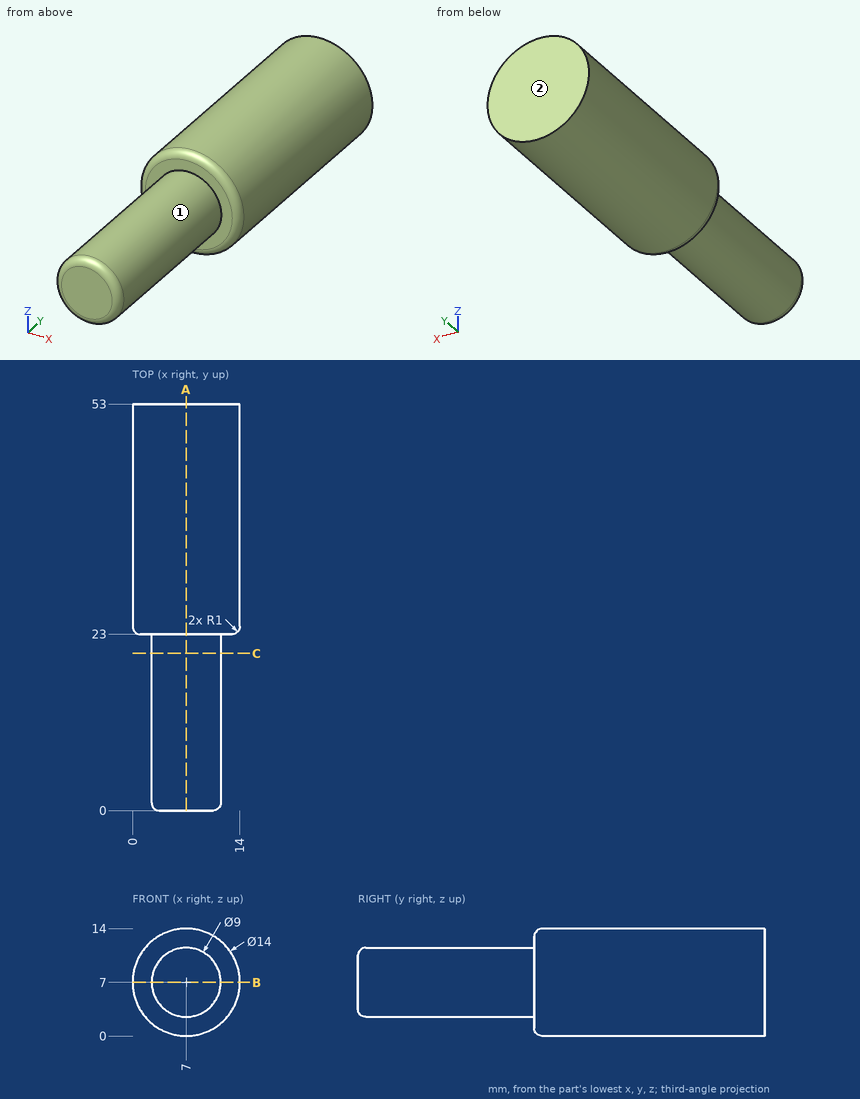
Part print with two shaded views. Sizes in mm from the minimum x, y, z corner. A direction names the side the tool comes from. Round coordinates to 2 decimals unless told otherwise and drop trailing zeros. Order: outer loops, then holes, each group sorted by start corner. A loop starts at its lowest first (then second) coordinate and runs counter-clockwise, first axis right, second up. Notation, with made-up numbers: M -3,-36.75 L 18,-36.75 A23 ccw 18,-14.75 Z; hole C 67,62 d7. An arc over 180 degrees is marked long. Use CSV: the item, a comma, the result in double quotes.
Item 1: Probe probe 1 along Y at (x, z) = (8, 1.5); probe 2 along Y at (x, z) = (5.5, 10.25); probe 3 along Z at (x, y) = (12.75, 43). List the from-to ranges inside material, lowest first.
Worked answers:
probe 1,"23 to 53"
probe 2,"0 to 53"
probe 3,"3.01 to 10.99"
Item 2: Saw through at C-C (y = 20.5). List the corners of the cut face in (x, z).
Worked answers:
outline,"C 7,7 d9"
Item 3: Which spindle directions (+Z, -Z, +X, -X, +Y, -Y) get a long thin tool onto all of the face, cutting with end or side? Do the marked faces 1 and 2. Say none if no direction does.
Worked answers:
face 1,"-Y"
face 2,"+Z, -Z, +X, -X, +Y"
Item 4: Pin check, flat tips, straight feed: pin 1 (2 mm diameter, centred on y = 25.5, z = 4.5, fed in from +X); pin 2 (5 mm diameter, centred on x = 3.5, z = 1.5, fed in from -Y); pin 3 (1.5 mm diameter, centred on y = 46, z = 12.5, fed in from -X). Stop position of each tip, or through.
Worked answers:
pin 1,"x = 13.84"
pin 2,"y = 0.15"
pin 3,"x = 1.86"
Item 5: Saw through at B-B (z = 7). List the corners of the cut face in (x, y).
Worked answers:
outline,"M 0,24 A1 ccw 1,23 L 2.5,23 L 2.5,1 A1 ccw 3.5,0 L 10.5,0 A1 ccw 11.5,1 L 11.5,23 L 13,23 A1 ccw 14,24 L 14,53 L 0,53 Z"
Item 6: Saw through at A-A (x = 7). List the corners of the cut face in (y, z), plus the area to 3 significant figures.
Worked answers:
outline,"M 0,3.5 A1 ccw 1,2.5 L 23,2.5 L 23,1 A1 ccw 24,0 L 53,0 L 53,14 L 24,14 A1 ccw 23,13 L 23,11.5 L 1,11.5 A1 ccw 0,10.5 Z"
area,"626 mm²"
